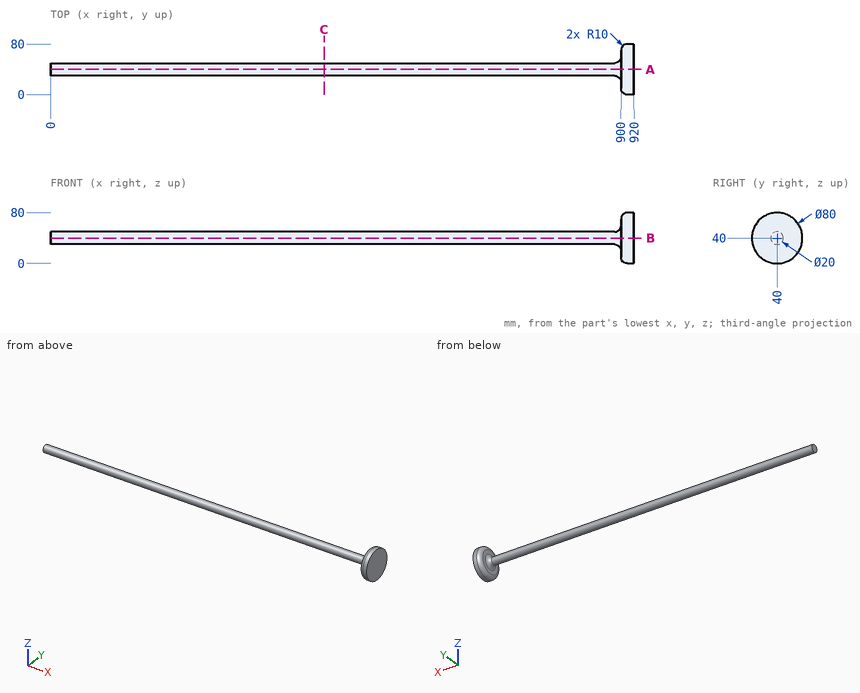
Could you check a few things on this drawing? It's one solid part, dimensions in mm from its lowest x, y, z. Give positions to 0.01 mm unless a question says otherwise; leave off trailing zeros. Loops run counter-clockwise (first coordinate to the right, second up) from the corner with the lowest first, then second, coordinate; pieces in that order, holes last. Notation, with made-up numbers: M 85.5,70 L 92.5,70 A22 cw 92.5,94 Z; hole C -23,19.5 d4. An arc over 180 degrees is marked long. Return JSON: item names as keys, results as strings.
Item 1: Imagine slicing it at C-C on x = 431.5. List the corners of the cut face in (y, z) for me.
A:
{"outline": "C 40,40 d20"}
Item 2: I'm going to push flat-ended pins straight in: pin 1 Ø4 at (x, y) = (636, 34) entering from +Z; pin 2 Ø1.5 at (x, z) = (547, 28) entering from +Y. Where does each tip first touch, or does it pass through?
A:
{"pin 1": "stops at z = 49.17", "pin 2": "passes through"}
Item 3: Please list where these lines run through material, in increasing order: line 1 (X direction, y = 56.5, z = 16); line 2 (Z direction, x = 759.5, y = 39); line 3 (X direction, y = 50, z = 27).
A:
{"line 1": "x = 900 to 920", "line 2": "z = 30.05 to 49.95", "line 3": "x = 899.33 to 920"}
Item 4: Imagine slicing it at A-A on y = 40. List the corners of the cut face in (x, z) for me.
A:
{"outline": "M 0,30 L 890,30 A10 cw 900,20 L 900,10 A10 ccw 910,0 L 920,0 L 920,80 L 910,80 A10 ccw 900,70 L 900,60 A10 cw 890,50 L 0,50 Z"}
